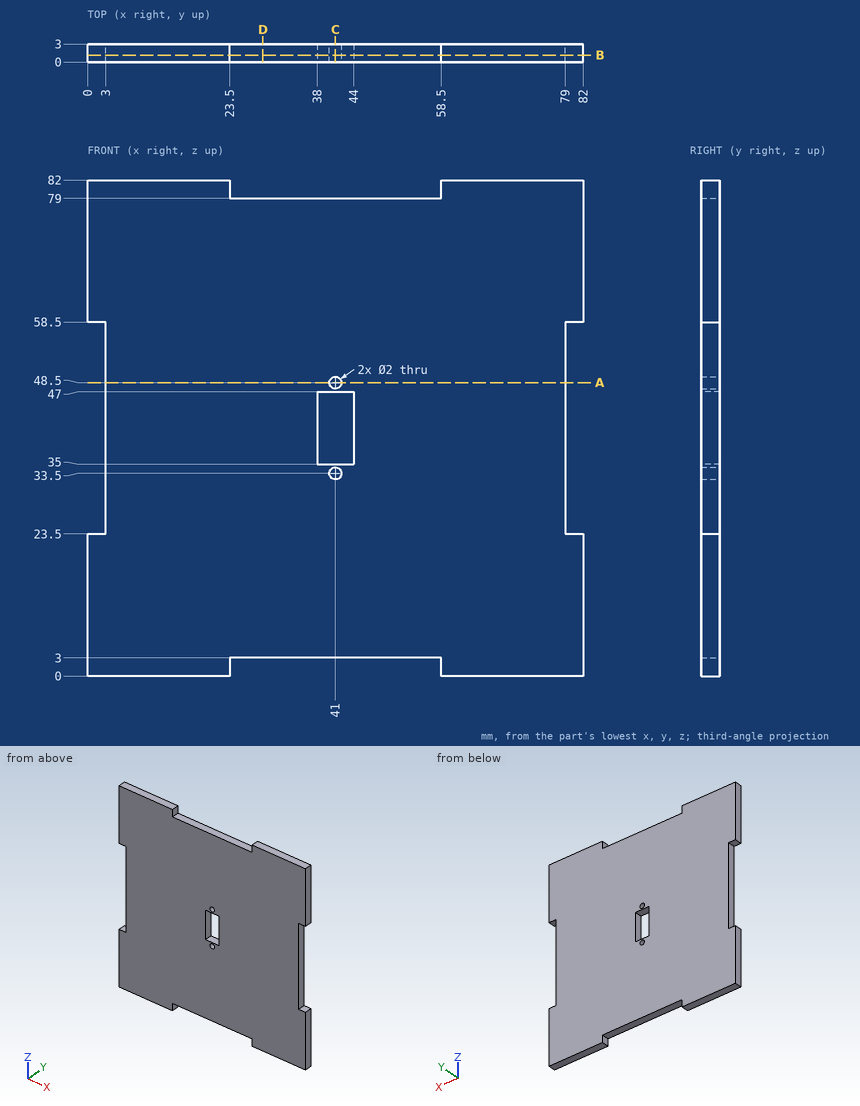
Here's the drawing with two shaded views (mm, measured from the low corner). I have some questions. Give positions to 0.01 mm unless a question says otherwise; leave off trailing zeros. Write each loop counter-clockwise with the first axis right and the second up, starting at its lowest first coordinate (ties: lowest second). Pieces come first, ordered by that corner, then holes. Notation, with made-up numbers: (64.25, -31) -> (69.25, -31) arc R33 ccw to (69.25, -2) -> close; hole circle Ø2 at (22.25, 77). An arc over 180 degrees is marked (long way). One line per item, written item: value.
Q1. Imagine slicing it at A-A on z = 48.5. Please give me the cut outline in (x, y).
Results found:
outline: (3, 0) -> (40, 0) -> (40, 3) -> (3, 3) -> close; (42, 0) -> (79, 0) -> (79, 3) -> (42, 3) -> close
Q2. Imagine slicing it at C-C on x = 41. Please give me the cut outline in (y, z).
Results found:
outline: (0, 3) -> (3, 3) -> (3, 32.5) -> (0, 32.5) -> close; (0, 34.5) -> (3, 34.5) -> (3, 35) -> (0, 35) -> close; (0, 47) -> (3, 47) -> (3, 47.5) -> (0, 47.5) -> close; (0, 49.5) -> (3, 49.5) -> (3, 79) -> (0, 79) -> close
Q3. Imagine slicing it at D-D on x = 29. Please give me the cut outline in (y, z).
Results found:
outline: (0, 3) -> (3, 3) -> (3, 79) -> (0, 79) -> close
Q4. Imagine slicing it at B-B on y = 1.15. Please give me the cut outline in (x, z).
Results found:
outline: (0, 0) -> (23.5, 0) -> (23.5, 3) -> (58.5, 3) -> (58.5, 0) -> (82, 0) -> (82, 23.5) -> (79, 23.5) -> (79, 58.5) -> (82, 58.5) -> (82, 82) -> (58.5, 82) -> (58.5, 79) -> (23.5, 79) -> (23.5, 82) -> (0, 82) -> (0, 58.5) -> (3, 58.5) -> (3, 23.5) -> (0, 23.5) -> close; hole (38, 35) -> (44, 35) -> (44, 47) -> (38, 47) -> close; hole circle Ø2 at (41, 33.5); hole circle Ø2 at (41, 48.5)
Q5. For P1, Ø0.9, axis at x = 48, y = 1.5, coming from the +Z side; P2, Ø1.5, axis at y = 1.5, z = 48.5, coming from the +X side; P3, Ø1.8, axis at x = 41, z = 48.5, coming from the +Y side; P4, Ø1.5, axis at x = 41.5, y = 2, coming from the -Z side, each with a flat end and sliding along its axis, tell me the tip position at first contact or that it passes through.
Results found:
P1: stops at z = 79
P2: stops at x = 79
P3: passes through
P4: stops at z = 3
Q6. Please list where these lines run through material, in increasing order: line 1 (Z direction, x = 41, y = 1.9); line 2 (X direction, y = 2.2, z = 33.5); line 3 (X direction, y = 1.45, z = 24). Write a range as [from, to].
Results found:
line 1: z = [3, 32.5], [34.5, 35], [47, 47.5], [49.5, 79]
line 2: x = [3, 40], [42, 79]
line 3: x = [3, 79]
